Build history of the part. All positions in model axes, mm. A direction names the side the tool comes from. Give positions to 0.01 mm unless a question says otherwise; leave off trailing zeros. Order: outer loops, then holes, each group sorted by start corner. A loop starts at its lowest first (then second) coordinate and runs counter-clockwise, first axis right, second up. Notation, with made-up numbers: (67, 80) - (99, 80) arc R13 ccw to (99, 99) - close; hole circle Ø10 at (88.5, 38.25). An arc over 180 degrees is marked (long way). Use a Markdown table: item, result.
from build123d import *

# Parameters (mm, degrees)
SKETCH3_R           = 4
BOSS_EXTRUDE1_DEPTH = 15
BOSS_EXTRUDE2_DEPTH = 60
FILLET1_R           = 1
SKETCH6_R           = 3.4
CUT_EXTRUDE1_DEPTH  = 116.10446612
SKETCH7_R           = 4
CUT_EXTRUDE2_DEPTH  = 116.10446612
CUT_EXTRUDE3_START  = -6
SKETCH8_R           = 7
CUT_EXTRUDE3_DEPTH  = 110.10446612
BOSS_EXTRUDE3_DEPTH = 15


with BuildPart() as part:
    # Sketch3 → Boss-Extrude1 (new body)
    with BuildSketch(Plane(origin=(0, 0, 0), x_dir=(1, 0, 0), z_dir=(0, 1, 0))):
        with BuildLine():
            ThreePointArc((52.056720354, -14.858327678), (65, 0), (52.056720354, 14.858327678))
            ThreePointArc((52.056720354, 14.858327678), (15.768189382, 27.311305152), (-13.16067095, 52.511606103))
            ThreePointArc((-13.16067095, 52.511606103), (-32.5, 56.291651246), (-38.896049404, 37.653278425))
            ThreePointArc((-38.896049404, 37.653278425), (-31.536378763, 0), (-38.896049404, -37.653278425))
            ThreePointArc((-38.896049404, -37.653278425), (-32.5, -56.291651246), (-13.16067095, -52.511606103))
            ThreePointArc((-13.16067095, -52.511606103), (15.768189382, -27.311305152), (52.056720354, -14.858327678))
        make_face()
        with Locations(Location((-25, 43.301270189, 0), (0, 0, 270))):
            Circle(SKETCH3_R, mode=Mode.SUBTRACT)
        with Locations(Location((-25, -43.301270189, 0), (0, 0, 270))):
            Circle(SKETCH3_R, mode=Mode.SUBTRACT)
        with Locations(Location((50, 0, 0), (0, 0, 270))):
            Circle(SKETCH3_R, mode=Mode.SUBTRACT)
        with BuildLine():
            Line((18.7, 4), (14.456832295, 4))
            ThreePointArc((14.456832295, 4), (-15, 0), (14.456832295, -4))
            Line((14.456832295, -4), (18.7, -4))
            Line((18.7, -4), (18.7, 4))
        make_face(mode=Mode.SUBTRACT)
    extrude(amount=BOSS_EXTRUDE1_DEPTH)

    # Sketch4 → Boss-Extrude2 (add)
    with BuildSketch(Plane(origin=(0, 15, 0), x_dir=(1, 0, 0), z_dir=(0, 1, 0))):
        with BuildLine():
            Line((18.7, -4), (14.456832295, -4))
            ThreePointArc((14.456832295, -4), (-1.271711896, -14.945994408), (-14.924811557, -1.5))
            Line((-14.924811557, -1.5), (-29.962476533, -1.5))
            ThreePointArc((-29.962476533, -1.5), (0.750234632, -29.990617666), (30, 0))
            ThreePointArc((30, 0), (0.750234632, 29.990617666), (-29.962476533, 1.5))
            Line((-29.962476533, 1.5), (-14.924811557, 1.5))
            ThreePointArc((-14.924811557, 1.5), (-1.271711896, 14.945994408), (14.456832295, 4))
            Line((14.456832295, 4), (18.7, 4))
            Line((18.7, 4), (18.7, -4))
        make_face()
    extrude(amount=BOSS_EXTRUDE2_DEPTH)

    # Fillet1
    fillet1_edges = [part.edges().sort_by_distance(p)[0] for p in [
        (30, 15, 0),
    ]]
    fillet(fillet1_edges, radius=FILLET1_R)

    # Sketch6 → Cut-Extrude1 (cut, through all)
    with BuildSketch(Plane.XY):
        with Locations(Location((-22.443644045, 65, 0), (0, 0, 180))):
            Circle(SKETCH6_R)
        with Locations(Location((-22.443644045, 45, 0), (0, 0, 180))):
            Circle(SKETCH6_R)
    extrude(amount=CUT_EXTRUDE1_DEPTH, mode=Mode.SUBTRACT)

    # Sketch7 → Cut-Extrude2 (cut, through all)
    with BuildSketch(Plane.XY):
        with Locations((-22.443644045, 65)):
            Circle(SKETCH7_R)
        with Locations((-22.443644045, 45)):
            Circle(SKETCH7_R)
    extrude(amount=-CUT_EXTRUDE2_DEPTH, mode=Mode.SUBTRACT)

    # Sketch8 → Cut-Extrude3 (cut, through all)
    with BuildSketch(Plane.XY.offset(CUT_EXTRUDE3_START)):
        with Locations((-22.443644045, 65)):
            Circle(SKETCH8_R)
        with Locations((-22.443644045, 45)):
            Circle(SKETCH8_R)
    extrude(amount=-CUT_EXTRUDE3_DEPTH, mode=Mode.SUBTRACT)

    # Sketch9 → Boss-Extrude3 (add)
    with BuildSketch(Plane(origin=(0, 0, 0), x_dir=(1, 0, 0), z_dir=(0, 1, 0))):
        with BuildLine():
            ThreePointArc((-38.896049404, 37.653278425), (-39.187845088, 48.170053586), (-32.499996308, 56.291653378))
            ThreePointArc((-32.499996308, 56.291653378), (-65, 1.908e-06), (-32.499999613, -56.29165147))
            ThreePointArc((-32.499999613, -56.29165147), (-39.187845707, -48.170051781), (-38.896049404, -37.653278425))
            ThreePointArc((-38.896049404, -37.653278425), (-31.536378763, 0), (-38.896049404, 37.653278425))
        make_face()
        with BuildLine():
            ThreePointArc((52.056720354, 14.858327678), (61.310411251, 9.85264418), (65, 0))
            ThreePointArc((65, 0), (32.500001846, 56.29165018), (-32.499996308, 56.291653378))
            ThreePointArc((-32.499996308, 56.291653378), (-22.122563378, 58.022695341), (-13.16067095, 52.511606103))
            ThreePointArc((-13.16067095, 52.511606103), (15.768189382, 27.311305152), (52.056720354, 14.858327678))
        make_face()
        with BuildLine():
            ThreePointArc((-32.499999613, -56.29165147), (32.500000194, -56.291651134), (65, 0))
            ThreePointArc((65, 0), (61.310411251, -9.85264418), (52.056720354, -14.858327678))
            ThreePointArc((52.056720354, -14.858327678), (15.768189382, -27.311305152), (-13.16067095, -52.511606103))
            ThreePointArc((-13.16067095, -52.511606103), (-22.122565251, -58.022695707), (-32.499999613, -56.29165147))
        make_face()
    extrude(amount=BOSS_EXTRUDE3_DEPTH)


solid = part.part
1) Wall check: line 1 (X direction, y = 5.75, z = 0); line 2 (Z direction, x = 0, y = 8.5); line 3 (Z direction, x = -0.5, y = 35.5). Give the ranges that are in metal, low to high. Write a range as from..to.
Computed:
| item | result |
|---|---|
| line 1 | x = -65..-15, 18.7..46, 54..65 |
| line 2 | z = -65..-15, 15..65 |
| line 3 | z = -30..-14.99, 14.99..30 |
2) Slice it at A-A (y = 11.5). Write the cut outline in (x, z), and give its area (3 significant figures).
Computed:
| item | result |
|---|---|
| outline | circle Ø130 at (0, 0); hole circle Ø8 at (-25, -43.3); hole circle Ø8 at (-25, 43.3); hole (14.46, -4) - (18.7, -4) - (18.7, 4) - (14.46, 4) arc R15 ccw (long way) to start; hole circle Ø8 at (50, 0) |
| area | 12,400 mm² |
3) Slice it at B-B (y = 20.5). Write the cut outline in (x, z), and give its area (3 significant figures).
Computed:
| item | result |
|---|---|
| outline | (-29.96, -1.5) arc R30 ccw (long way) to (-29.96, 1.5) - (-14.92, 1.5) arc R15 cw to (14.46, 4) - (18.7, 4) - (18.7, -4) - (14.46, -4) arc R15 cw to (-14.92, -1.5) - close |
| area | 2,040 mm² |
4) Two-plate mould, pull along X, no slides. Class faces 6 (the flat face through (6, 75, -14)), 7 (the cylindrical face through (-19.047, 44.851, 9.783)): +X half, -X half, draft (parallel to the pull), parting line (faces both ways), or undercut.
Computed:
| item | result |
|---|---|
| face 6 | draft |
| face 7 | undercut |
5) Tool access for faces 1 (the cylindrical face through (-19.047, 64.851, 9.783)), 2 (the flat face through (-19, 62, -6)), 3 (the flat face through (-27, 45, -1.5)), 4 (the flat face through (-15.4, 15, -0.9)), 5 (the flat face through (18.7, 37, 0)): list every direction of +Z, -Z, +X, -X, +Y, -Y with a clear straight run to the whole face (end or side of a thin tool).
Computed:
| item | result |
|---|---|
| face 1 | +Z, -Z |
| face 2 | -Z |
| face 3 | -X, +Y |
| face 4 | +Y |
| face 5 | +Y, -Y |
6) Pin check, flat tips, straight feed: P1, Ø4, axis at x = 35, z = 9, coming from the +Y side; P2, Ø8, axis at x = -22.44, y = 45, coming from the +Z side; P3, Ø9, axis at x = 50, z = 0, coming from the -Y side; P4, Ø7, axis at x = -25, z = -43.3, coming from the -Y side. Stop position of each tip, or through.
Computed:
| item | result |
|---|---|
| P1 | stops at y = 15 |
| P2 | stops at z = 23.66 |
| P3 | stops at y = 0 |
| P4 | passes through |
7) Slice it at C-C (z = 35). Write the cut outline in (x, y), and give its area (3 significant figures).
Computed:
| item | result |
|---|---|
| outline | (-54.77, 0) - (54.77, 0) - (54.77, 15) - (-54.77, 15) - close |
| area | 1,640 mm² |
